from build123d import *

# Parameters (mm, degrees)
VENTED_LID_RISER_PROFILE_W = 145
VENTED_LID_RISER_PROFILE_H = 55
VENTED_LID_RISER_PROFILE_R = 2.1
VENTED_LID_RISER_DEPTH     = 3


with BuildPart() as part:
    # Vented lid riser profile → Vented lid riser (new body)
    with BuildSketch(Plane.XY):
        with Locations((-18.5, 79.5)):
            Rectangle(VENTED_LID_RISER_PROFILE_W, VENTED_LID_RISER_PROFILE_H)
        with Locations((-51, 61)):
            Circle(VENTED_LID_RISER_PROFILE_R, mode=Mode.SUBTRACT)
        with Locations((45, 61)):
            Circle(VENTED_LID_RISER_PROFILE_R, mode=Mode.SUBTRACT)
        with BuildLine():
            Line((-72.5, 79), (-41.5, 79))
            ThreePointArc((-41.5, 79), (-38.5, 82), (-41.5, 85))
            Line((-41.5, 85), (-72.5, 85))
            ThreePointArc((-72.5, 85), (-75.5, 82), (-72.5, 79))
        make_face(mode=Mode.SUBTRACT)
        with BuildLine():
            Line((-30.5, 79), (0.5, 79))
            ThreePointArc((0.5, 79), (3.5, 82), (0.5, 85))
            Line((0.5, 85), (-30.5, 85))
            ThreePointArc((-30.5, 85), (-33.5, 82), (-30.5, 79))
        make_face(mode=Mode.SUBTRACT)
        with BuildLine():
            Line((11.5, 79), (42.5, 79))
            ThreePointArc((42.5, 79), (45.5, 82), (42.5, 85))
            Line((42.5, 85), (11.5, 85))
            ThreePointArc((11.5, 85), (8.5, 82), (11.5, 79))
        make_face(mode=Mode.SUBTRACT)
    extrude(amount=VENTED_LID_RISER_DEPTH)


solid = part.part
CAD build for the part. Positions are in the model's coordinates, mm. A direction names the side the tool comes from. Round coordinates to 2 decimals unless told otherwise and drop trailing zeros. Write each loop counter-clockwise with the first axis right and the second up, starting at its lowest first coordinate (ties: lowest second). Pieces come first, ordered by that corner, then holes.
(1) Mould opens along X. For faces 3 (the face through (-38.5, 81.9, 1.5)), 4 (the face through (-91, 79, 1)), 5 (the face through (-20, 86, 0)) say: pulls with the +X half, pulls with the -X half, needs draft (parallel to the pull), parting line crosses it, or undercut.
(2) Slice it at D-D, the plane y = 82. Write the cut outline in (x, z).
(3) 3-axis set-ups, long thin cutter, end or side, ignore diameter. For faces 1 (the face through (-20, 86, 3)), 2 (the face through (-75.5, 82.1, 1.5)): which of +Z, -Z, +X, -X, +Y, -Y reach the whole face in a straight line?
(4) Drop a flat-ended pin along its axis: P1, Ø4, axis at x = 45, y = 61, coming from the +Z side. Give the stop position or say it passes through.
(5) Probe line 1 along Y through (x, z) = (-51, 1.1); line 2 along Y through (x, z) = (-56, 1); line 3 along Y through (x, z) = (45, 1.35). List the from-to ranges inside material, lowest first.
(6) Slice it at B-B, the plane x = -51. Write the cut outline in (y, z), and give its area (3 significant figures).
(7) Slice it at A-A, the plane y = 61. Write the cut outline in (x, z), and give its area (3 significant figures).
(8) Slice it at C-C, the plane z = 0.9. Write the cut outline in (x, y).
From the geometry:
1. face 3: undercut
1. face 4: pulls with the -X half
1. face 5: needs draft
2. outline: (-91, 0) - (-75.5, 0) - (-75.5, 3) - (-91, 3) - close; (-38.5, 0) - (-33.5, 0) - (-33.5, 3) - (-38.5, 3) - close; (3.5, 0) - (8.5, 0) - (8.5, 3) - (3.5, 3) - close; (45.5, 0) - (54, 0) - (54, 3) - (45.5, 3) - close
3. face 1: +Z, +X, -X, +Y, -Y
3. face 2: +Z, -Z
4. P1: passes through
5. line 1: y = 52 to 58.9, 63.1 to 79, 85 to 107
5. line 2: y = 52 to 79, 85 to 107
5. line 3: y = 52 to 58.9, 63.1 to 80.34, 83.66 to 107
6. outline: (52, 0) - (58.9, 0) - (58.9, 3) - (52, 3) - close; (63.1, 0) - (79, 0) - (79, 3) - (63.1, 3) - close; (85, 0) - (107, 0) - (107, 3) - (85, 3) - close
6. area: 134 mm2
7. outline: (-91, 0) - (-53.1, 0) - (-53.1, 3) - (-91, 3) - close; (-48.9, 0) - (42.9, 0) - (42.9, 3) - (-48.9, 3) - close; (47.1, 0) - (54, 0) - (54, 3) - (47.1, 3) - close
7. area: 410 mm2
8. outline: (-91, 52) - (54, 52) - (54, 107) - (-91, 107) - close; hole (-72.5, 79) - (-41.5, 79) arc R3 ccw to (-41.5, 85) - (-72.5, 85) arc R3 ccw to start; hole circle Ø4.2 at (-51, 61); hole (-30.5, 79) - (0.5, 79) arc R3 ccw to (0.5, 85) - (-30.5, 85) arc R3 ccw to start; hole (11.5, 79) - (42.5, 79) arc R3 ccw to (42.5, 85) - (11.5, 85) arc R3 ccw to start; hole circle Ø4.2 at (45, 61)
